from build123d import *

# Parameters (mm, degrees)
SZKIC1_R                    = 67
SZKIC1_R_2                  = 3
DODANIE_WYCI_GNI_CIE1_DEPTH = 5
SZKIC2_R                    = 1.937371164
WYTNIJ_WYCI_GNI_CIE1_DEPTH  = 2


with BuildPart() as part:
    # Szkic1 → Dodanie-wyciągnięcie1 (new body)
    with BuildSketch(Plane.XY):
        Circle(SZKIC1_R)
        with Locations((0, 25)):
            Circle(SZKIC1_R_2, mode=Mode.SUBTRACT)
        with Locations((25, 0)):
            Circle(SZKIC1_R_2, mode=Mode.SUBTRACT)
        with Locations((0, -25)):
            Circle(SZKIC1_R_2, mode=Mode.SUBTRACT)
        with Locations((-25, 0)):
            Circle(SZKIC1_R_2, mode=Mode.SUBTRACT)
    extrude(amount=DODANIE_WYCI_GNI_CIE1_DEPTH)

    # Szkic2 → Wytnij-wyciągnięcie1 (cut)
    with BuildSketch(Plane.XY.offset(5)):
        with BuildLine():
            Line((6.015596419, 12.825090242), (-16.98777971, 12.825090242))
            add(Edge.make_bspline(
                [(-16.98777971, 12.825090242), (-21.398431669, 13.157388334), (-22.546113217, 2.558365481), (-11.828245601, 3.533872092), (-9.796666854, 8.186074774), (-6.590160082, 8.194882462)],
                knots=[0, 0, 0, 0, 0.432020753, 0.673133157, 1, 1, 1, 1], degree=3))
            Line((-6.590160082, 8.194882462), (6.347109239, 8.194882462))
            add(Edge.make_bspline(
                [(6.750985333, 2.833348247), (8.366457692, 3.074986228), (9.070388327, 5.597763216), (7.624972799, 7.999760841), (6.347109239, 8.194882462)],
                knots=[0, 0, 0, 0, 0.494793037, 1, 1, 1, 1], degree=3))
            Line((6.750985333, 2.833348247), (-6.742018824, 2.833348247))
            add(Edge.make_bspline(
                [(-6.015596419, -12.825090242), (-10.545778612, -13.3417132), (-16.414760064, -4.631679813), (-10.491978135, 2.966309296), (-6.742018824, 2.833348247)],
                knots=[0, 0, 0, 0, 0.544342745, 1, 1, 1, 1], degree=3))
            Line((-6.015596419, -12.825090242), (16.98777971, -12.825090242))
            add(Edge.make_bspline(
                [(16.98777971, -12.825090242), (21.398431669, -13.157388334), (22.546113217, -2.558365481), (11.828245601, -3.533872092), (9.796666854, -8.186074774), (6.590160082, -8.194882462)],
                knots=[0, 0, 0, 0, 0.432020753, 0.673133157, 1, 1, 1, 1], degree=3))
            Line((6.590160082, -8.194882462), (-6.347109239, -8.194882462))
            add(Edge.make_bspline(
                [(-6.742018824, -2.341525215), (-8.383912674, -2.639536282), (-9.106573397, -5.485782084), (-7.635691285, -7.991138773), (-6.347109239, -8.194882462)],
                knots=[0, 0, 0, 0, 0.526459521, 1, 1, 1, 1], degree=3))
            Line((-6.742018824, -2.341525215), (6.750985333, -2.341525215))
            add(Edge.make_bspline(
                [(6.015596419, 12.825090242), (10.510890039, 13.359942568), (16.495321184, 4.672671746), (10.416213029, -2.612973757), (6.750985333, -2.341525215)],
                knots=[0, 0, 0, 0, 0.552476507, 1, 1, 1, 1], degree=3))
        make_face()
        with Locations((-16.245257119, 8.194882462)):
            Circle(SZKIC2_R, mode=Mode.SUBTRACT)
        with Locations((16.245257119, -8.194882462)):
            Circle(SZKIC2_R, mode=Mode.SUBTRACT)
    extrude(amount=-WYTNIJ_WYCI_GNI_CIE1_DEPTH, mode=Mode.SUBTRACT)


solid = part.part
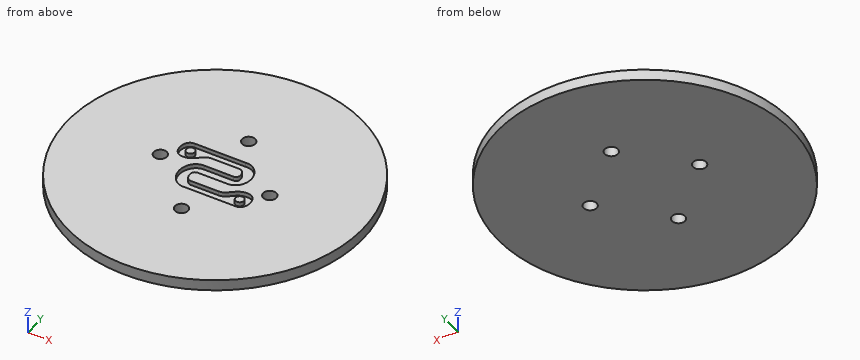
For this review, take the finished solid that the model builds, in its own axes (mm). Round coordinates to 2 decimals unless told otherwise and drop trailing zeros. Order: outer loops, then holes, each group sorted by start corner. A loop starts at its lowest first (then second) coordinate and runs counter-clockwise, first axis right, second up. Notation, with made-up numbers: M 65,75 L 88,75 A25 cw 88,99 Z; hole C -29,39 d3. An arc over 180 degrees is marked long. Use a Markdown table: item, result. Add a question column.
Item 1: To check wall thickness, follow line 1 along Y through (x, z) = (0, 3.7); line 2 along Y through (x, z) = (0, 1.25); line 3 along Y through (x, z) = (25, 3.7). State the ranges of each line that lie inside material, in increasing order.
Item 2: Add section A-A, the plane x = 0. Give the boundary of the cut face in (y, z), then the cut area to 3 significant figures.
Item 3: Insertion check: pin 1 (0.6 mm diameter, centred on x = 3, z = 4, fed in from -Y); pin 2 (9.5 mm diameter, centred on x = 25, y = 0, fed in from -Z); pin 3 (3 mm diameter, centred on x = -2, z = 0.5, fed in from +Y); pin 4 (1 mm diameter, centred on y = 30.5, z = 2.5, fed in from +X). Each pin has a flat end and moves straight along its axis. Give the tip position at first contact, or say it passes through.
Item 4: Add section C-C, the plane y = -25. Give the boundary of the cut face in (x, z), then the cut area to 3 significant figures.
Item 5: Add section D-D, the plane y = 34.5. Give the boundary of the cut face in (x, z).
Item 6: Add section B-B, the plane x = -24.5. Give the boundary of the cut face in (y, z).
Geometry results:
| question | item | result |
|---|---|---|
| 1 | line 1 | y = -67 to -28, -22 to -12.83, -8.19 to -2.34, 2.83 to 8.19, 12.83 to 22, 28 to 67 |
| 1 | line 2 | y = -67 to -28, -22 to 22, 28 to 67 |
| 1 | line 3 | y = -62.16 to -3, 3 to 62.16 |
| 2 | outline | M -67,0 L -28,0 L -28,5 L -67,5 Z; M -22,0 L 22,0 L 22,5 L 12.83,5 L 12.83,3 L 8.19,3 L 8.19,5 L 2.83,5 L 2.83,3 L -2.34,3 L -2.34,5 L -8.19,5 L -8.19,3 L -12.83,3 L -12.83,5 L -22,5 Z; M 28,0 L 67,0 L 67,5 L 28,5 Z |
| 2 | area | 581 mm² |
| 3 | pin 1 | stops at y = -66.95 |
| 3 | pin 2 | stops at z = 0 |
| 3 | pin 3 | stops at y = 67 |
| 3 | pin 4 | stops at x = 59.91 |
| 4 | outline | M -62.16,0 L -3,0 L -3,5 L -62.16,5 Z; M 3,0 L 62.16,0 L 62.16,5 L 3,5 Z |
| 4 | area | 592 mm² |
| 5 | outline | M -57.43,0 L 57.43,0 L 57.43,5 L -57.43,5 Z |
| 6 | outline | M -62.36,0 L -2.96,0 L -2.96,5 L -62.36,5 Z; M 2.96,0 L 62.36,0 L 62.36,5 L 2.96,5 Z |
